```python
from build123d import *

# Parameters (mm, degrees)
F1_DEPTH = 100
F2_R     = 1.5
F3_DEPTH = 8
F4_R     = 1.875
F5_DEPTH = 9
F6_R     = 1.875
F7_DEPTH = 9


with BuildPart() as f1:
    # F0 (on Right) → F1 (new body)
    with BuildSketch(Plane.YZ):
        Polygon((21.477706, -37.121146), (21.477706, 53.878854), (15.477706, 53.878854), (15.477706, -31.121146), (5.477706, -31.121146), (5.477706, -16.121146), (-0.522294, -16.121146), (-0.522294, -37.121146), align=None)
    extrude(amount=F1_DEPTH)

    # F2 (on face) → F3 (join)
    with BuildSketch(Plane.YZ.offset(100)):
        with Locations((18.477706, 43.878854)):
            Circle(F2_R)
        with Locations((18.477706, 23.878854)):
            Circle(F2_R)
        with Locations((18.477706, -7.121146)):
            Circle(F2_R)
        with Locations((18.477706, -27.121146)):
            Circle(F2_R)
    extrude(amount=F3_DEPTH)

    # F4 (on face) → F5 (cut)
    with BuildSketch(Plane(origin=(0, 0, 0), x_dir=(0, -1, 0), z_dir=(-1, 0, 0))):
        with Locations((-18.477706, 23.878854)):
            Circle(F4_R)
        with Locations((-18.477706, 43.878854)):
            Circle(F4_R)
        with Locations((-18.477706, -7.121146)):
            Circle(F4_R)
        with Locations((-18.477706, -27.121146)):
            Circle(F4_R)
    extrude(amount=-F5_DEPTH, mode=Mode.SUBTRACT)

    # F6 (on face) → F7 (cut)
    with BuildSketch(Plane(origin=(0, 21.477706, 0), x_dir=(-1, 0, 0), z_dir=(0, 1, 0))):
        with Locations((-80, -34.121146)):
            Circle(F6_R)
        with Locations((-60, -34.121146)):
            Circle(F6_R)
        with Locations((-40, -34.121146)):
            Circle(F6_R)
        with Locations((-20, -34.121146)):
            Circle(F6_R)
    extrude(amount=-F7_DEPTH, mode=Mode.SUBTRACT)


solid = f1.part
```
For this review, take the finished solid that the model builds, in its own axes (mm). A direction names the side the tool comes from. Round coordinates to 2 decimals unless told otherwise and drop trailing zeros. Loops run counter-clockwise (first coordinate to the right, second up) from the corner with the lowest first, then second, coordinate; pieces in that order, holes last.
(1) Wall thickness on line 1 along Z through (x, y) = (80, 18); line 2 along X through (y, z) = (16, -1); line 3 along Z through (x, y) = (74, 1.5): over which ranges is each line inside the solid? List them lowest first.
Returned:
line 1: z = -37.12 to -36, -32.25 to 53.88
line 2: x = 0 to 100
line 3: z = -37.12 to -16.12
(2) We need section A-A (x = 49.5). Give the boundary of the cut face in (y, z).
Returned:
outline: (-0.52, -37.12) - (21.48, -37.12) - (21.48, 53.88) - (15.48, 53.88) - (15.48, -31.12) - (5.48, -31.12) - (5.48, -16.12) - (-0.52, -16.12) - close
(3) We need section C-C (z = 27). Give the boundary of the cut face in (x, y), plus the area to 3 significant figures.
Returned:
outline: (0, 15.48) - (100, 15.48) - (100, 21.48) - (0, 21.48) - close
area: 600 mm2
(4) Mouldability with a two-part tool opening along X and no side actions: class faces 1 (the flat face through (9, 19, -7)), 2 (the flat face through (100, 16, 2)), 3 (the cylindrical face through (60.41, 17.04, -35.95)) as released by +X, released by -X, zero draft, split by the parting line, or undercut.
Returned:
face 1: released by -X
face 2: released by +X
face 3: undercut
(5) We need section B-B (y = 14). Give the boundary of the cut face in (x, z) (3 decimals), plus the area to 3 significant figures.
Returned:
outline: (0, -37.121) - (100, -37.121) - (100, -31.121) - (0, -31.121) - close; hole circle Ø3.75 at (20, -34.121); hole circle Ø3.75 at (40, -34.121); hole circle Ø3.75 at (60, -34.121); hole circle Ø3.75 at (80, -34.121)
area: 556 mm2
(6) We need section D-D (x = 80). Give the boundary of the cut face in (y, z), plus the area to 3 significant figures.
Returned:
outline: (-0.52, -37.12) - (21.48, -37.12) - (21.48, -36) - (12.48, -36) - (12.48, -32.25) - (21.48, -32.25) - (21.48, 53.88) - (15.48, 53.88) - (15.48, -31.12) - (5.48, -31.12) - (5.48, -16.12) - (-0.52, -16.12) - close
area: 698 mm2
(7) Clearance check with flat-ended pins moving along their axes: P1, Ø5, axis at x = 43, y = 5.5, coming from the +Z side; P2, Ø3, axis at x = 91, z = 24, coming from the -Y side; P3, Ø2, axis at x = 80, z = -34.12, coming from the +Y side. State where each tip first meets the part, or that it passes through.
Returned:
P1: stops at z = -16.12
P2: stops at y = 15.48
P3: stops at y = 12.48
(8) Tool access review of faces 4 (the flat face through (60, 12.478, -34)), 5 (the flat face through (9, 19, -27)), 6 (the cylindrical face through (103.94, 19.86, -7.7)): name each direction out of +Z, -Z, +X, -X, +Y, -Y from which nothing blocks a thin tool from reaching the whole face with its end or side.
Returned:
face 4: +Y
face 5: -X
face 6: +X
